Autodesk Inventor part; units mm, degrees
ref_plane "YZ Plane" through (0, 0, 0) normal (1, 0, 0) x (0, 1, 0)
ref_plane "XZ Plane" through (0, 0, 0) normal (0, 1, 0) x (-1, 0, 0)
ref_plane "XY Plane" through (0, 0, 0) normal (0, 0, 1) x (1, 0, 0)
sketch "Sketch1" plane through (0, 0, 0) normal (0, 0, 1) x (1, 0, 0)
  line L0 (0, 0) -> (25.4, 0)
  line L1 (25.4, 0) -> (25.4, 25.4)
  line L2 (25.4, 25.4) -> (0, 25.4)
  line L3 (0, 25.4) -> (0, 0)
  line L4 (3.175, 22.225) -> (22.225, 22.225)
  line L5 (22.225, 22.225) -> (22.225, 3.175)
  line L6 (22.225, 3.175) -> (3.175, 3.175)
  line L7 (3.175, 3.175) -> (3.175, 22.225)
  dimension "d0" = 25.4
  dimension "d1" = 25.4
  dimension "d2" = 3.175
extrude "Extrusion1" add sketch "Sketch1" along normal blind 914.4
sketch "Sketch2" plane through (0, 25.4, 0) normal (0, 1, 0) x (1, 0, 0)
  line L0 (0, 0) -> (25.4, 0) construction
  line L1 (12.7, 0) -> (12.7, -12.7) construction
  line L2 (12.7, -12.7) -> (12.7, -38.1) construction
  line L3 (12.7, -38.1) -> (12.7, -63.5) construction
  line L4 (0, 0) -> (0, -914.4) construction
  line L5 (0, 0) -> (0, -139.7) construction
  line L6 (0, -139.7) -> (25.4, -139.7) construction
  line L7 (12.7, -139.7) -> (12.7, -114.3) construction
  line L8 (12.7, -114.3) -> (12.7, -165.1) construction
  line L9 (0, -457.2) -> (25.4, -457.2) construction
  line L10 (25.4, 0) -> (25.4, -914.4) construction
  circle A0 centre (12.7, -139.7) radius 2.5797
  circle A1 centre (12.7, -114.3) radius 2.5797
  circle A2 centre (12.7, -165.1) radius 2.5797
  circle A3 centre (12.7, -63.5) radius 2.5797
  circle A4 centre (12.7, -38.1) radius 2.5797
  circle A5 centre (12.7, -12.7) radius 2.5797
  circle A6 centre (12.7, -774.7) radius 2.5797
  circle A7 centre (12.7, -800.1) radius 2.5797
  circle A8 centre (12.7, -749.3) radius 2.5797
  circle A9 centre (12.7, -850.9) radius 2.5797
  circle A10 centre (12.7, -876.3) radius 2.5797
  circle A11 centre (12.7, -901.7) radius 2.5797
  dimension "d5" = 12.7
  dimension "d6" = 25.4
  dimension "d7" = 25.4
  dimension "d8" = 139.7
  dimension "d9" = 25.4
  dimension "d10" = 50.8
  dimension "d11" = 5.1594
extrude "Extrusion2" cut sketch "Sketch2" against normal blind 914.4
properties part number "3ft 1x1"
Verification items for the finished model (mm, model axes). A direction names the side the tool comes from. Round coordinates to 2 decimals unless told otherwise and drop trailing zeros. Order: outer loops, then holes, each group sorted by start corner. A loop starts at its lowest first (then second) coordinate and runs counter-clockwise, first axis right, second up.
1. Thickness scan on L1, parallel to Y at x = 5.75, z = 67.5 (3 decimals); L2, parallel to X at y = 2.1, z = 165.1. Record the ranges inside material, lowest first.
Final values:
L1: y = 0 to 3.175, 22.225 to 25.4
L2: x = 0 to 10.12, 15.28 to 25.4
2. Access from +Z, -Z, +X, -X, +Y, -Y to the whole of each face (thin tool, end or side, straight path). Record for faces 1 (the flat face through (13, 25.4, 451)), 2 (the flat face through (3.175, 13, 451)).
Final values:
face 1: +Z, -Z, +X, -X, +Y
face 2: +Z, -Z
3. Go/stop test with flat-tipped pins: P1, Ø6.5, axis at x = 12.7, z = 774.7, coming from the -Y side; P2, Ø4, axis at x = 12.7, z = 901.7, coming from the -Y side. Record where each tip stops, or that it passes through.
Final values:
P1: stops at y = 0
P2: passes through
4. Release check for a two-part mould opening along X. For faces 3 (the flat face through (13, 3.175, 451)), 4 (the flat face through (22.225, 13, 451)), 5 (the flat face through (24, 13, 0)), 6 (the flat face through (0, 13, 451)) record: +X half, -X half, draft (parallel to the pull), parting line (faces both ways), or undercut.
Final values:
face 3: undercut
face 4: undercut
face 5: draft
face 6: -X half
5. Section check B-B on y = 14.25. Record the cut outline in (x, z) (3 decimals).
Final values:
outline: (0, 0) - (3.175, 0) - (3.175, 914.4) - (0, 914.4) - close; (22.225, 0) - (25.4, 0) - (25.4, 914.4) - (22.225, 914.4) - close
6. Section check A-A on z = 582.5. Record the cut outline in (x, y) (3 decimals).
Final values:
outline: (0, 0) - (25.4, 0) - (25.4, 25.4) - (0, 25.4) - close; hole (3.175, 3.175) - (22.225, 3.175) - (22.225, 22.225) - (3.175, 22.225) - close
